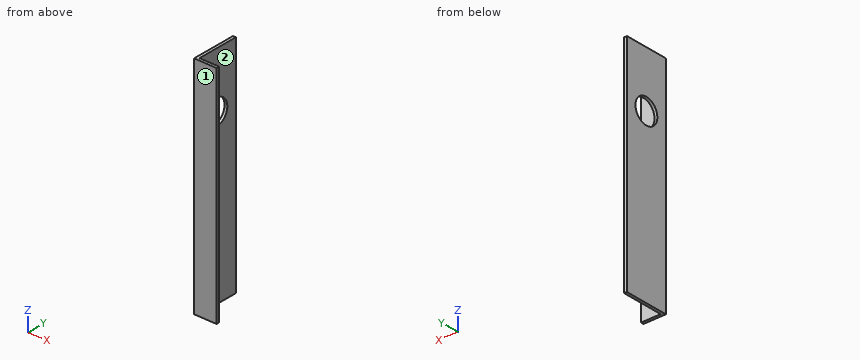
Autodesk Inventor part; units mm, degrees
ref_plane "YZ Plane" through (0, 0, 0) normal (1, 0, 0) x (0, 1, 0)
ref_plane "XZ Plane" through (0, 0, 0) normal (0, 1, 0) x (-1, 0, 0)
ref_plane "XY Plane" through (0, 0, 0) normal (0, 0, 1) x (1, 0, 0)
sketch "Sketch1" plane through (0, 0, 0) normal (0, 0, 1) x (1, 0, 0)
  line L0 (0, 0) -> (25.4, 0)
  line L1 (25.4, 0) -> (25.4, 3.175)
  line L2 (3.175, 50.8) -> (0, 50.8)
  line L3 (0, 50.8) -> (0, 0)
  line L4 (3.175, 50.8) -> (3.175, 3.175)
  line L5 (3.175, 3.175) -> (25.4, 3.175)
  dimension "d0" = 50.8
  dimension "d1" = 25.4
  dimension "d2" = 3.175
  dimension "d3" = 3.175
extrude "Extrusion1" add sketch "Sketch1" along normal blind 254
sketch "Sketch2" plane through (0, 0, 0) normal (-1, 0, 0) x (0, 0, 1)
  line L0 (0, 0) -> (254, 0)
  circle A0 centre (190.5, 25.4) radius 14.2875
  line L1 (254, 0) -> (254, 50.8)
  dimension "d6" = 28.575
  dimension "d8" = 25.4
  dimension "d11" = 63.5
extrude "Extrusion2" cut sketch "Sketch2" against normal through all
equation "\"d2\" = d3"
properties part number "8 ball bearing plate left"
Check sheet for the modelled part. Datum: model origin and axes. Units: mm. Face numbers are marked on the shaded views. A direction names the side the tool comes from. Round coordinates to 2 decimals unless told otherwise and drop trailing zeros. Loops run counter-clockwise (first coordinate to the right, second up) from the corner with the lowest first, then second, coordinate; pieces in that order, holes last. Notation, with made-up numbers: M 13.25,69.5 L 61.25,69.5 A15 cw 61.25,92.5 Z; hole C -4.5,56 d6. An arc over 180 degrees is marked long. One line per question, with ' | ' between items. Start each with the question number.
Item 1: Section check C-C (x = 16.75). Record the boundary of the cut face in (y, z) (3 decimals), and give its area (3 significant figures).
Item 2: Section check A-A (z = 190.5). Record the boundary of the cut face in (x, y) (1 decimal), and give its area (3 significant figures).
Item 3: Scan lines: probe 1 along Y at (x, z) = (1.65, 190.5); probe 2 along X at (y, z) = (18, 61.5) (3 decimals). Record each from-to range of solid material in increasing order.
Item 4: Section check B-B (y = 25.4). Record the boundary of the cut face in (x, z) (1 decimal).
Item 5: Set-up check for the marked faces 1 and 2: record each of +Z, -Z, +X, -X, +Y, -Y from which the full face is reachable in a straight line by a thin tool's end or side.
Item 6: Gauge pin test, flat ends, axial feed: pin 1 Ø2 at (y, z) = (20, 149.5) entering from +X (3 decimals); pin 2 Ø1.5 at (x, z) = (12, 119) entering from +Y (3 decimals). Record the tip position at first contact, or that the pin passes through.
Worked out:
1) outline: M 0,0 L 3.175,0 L 3.175,254 L 0,254 Z | area: 806 mm^2
2) outline: M 0,0 L 25.4,0 L 25.4,3.2 L 3.2,3.2 L 3.2,11.1 L 0,11.1 Z; M 0,39.7 L 3.2,39.7 L 3.2,50.8 L 0,50.8 Z | area: 141 mm^2
3) probe 1: 0 to 11.11, 39.69 to 50.8 | probe 2: 0 to 3.175
4) outline: M 0,0 L 3.2,0 L 3.2,176.2 L 0,176.2 Z; M 0,204.8 L 3.2,204.8 L 3.2,254 L 0,254 Z
5) face 1: +Z, -Z, +X, -X, -Y | face 2: +Z, -Z, +X, +Y
6) pin 1: x = 3.175 | pin 2: y = 3.175
